from build123d import *

# Parameters (mm, degrees)
SKETCH1_R                  = 75
BOSS_EXTRUDE1_DEPTH        = 5
SKETCH2_R                  = 75
SKETCH2_R_2                = 73
BOSS_EXTRUDE2_DEPTH        = 60
BOSS_EXTRUDE3_START        = -60
BOSS_EXTRUDE3_DEPTH        = 60
F_10_0MM_DOWEL_HOLE1_D     = 10
F_10_0MM_DOWEL_HOLE1_DEPTH = 5
F_10_0MM_DOWEL_HOLE1_TIP   = 3.004303095
CUT_EXTRUDE1_REACH         = 173.61
CUT_EXTRUDE1_END_RADIUS    = 75
SKETCH7_W                  = 66.452990904
SKETCH7_H                  = 16
CUT_EXTRUDE2_START         = -39
CUT_EXTRUDE2_DEPTH         = 39


with BuildPart() as part:
    # Sketch1 → Boss-Extrude1 (new body)
    with BuildSketch(Plane(origin=(0, 0, 0), x_dir=(1, 0, 0), z_dir=(0, 1, 0))):
        with Locations(Location((0, 0, 0), (0, 0, 270))):
            Circle(SKETCH1_R)
    extrude(amount=BOSS_EXTRUDE1_DEPTH)

    # Sketch2 → Boss-Extrude2 (add)
    with BuildSketch(Plane(origin=(0, 5, 0), x_dir=(1, 0, 0), z_dir=(0, 1, 0))):
        with Locations(Location((0, 0, 0), (0, 0, 270))):
            Circle(SKETCH2_R)
        with Locations(Location((0, 0, 0), (0, 0, 270))):
            Circle(SKETCH2_R_2, mode=Mode.SUBTRACT)
    extrude(amount=BOSS_EXTRUDE2_DEPTH)

    # Sketch3 → Boss-Extrude3 (add)
    with BuildSketch(Plane(origin=(0, 65, 0), x_dir=(1, 0, 0), z_dir=(0, 1, 0)).offset(BOSS_EXTRUDE3_START)):
        with BuildLine():
            ThreePointArc((26.551836095, 68), (0, 73), (-26.551836095, 68))
            Line((-26.551836095, 68), (26.551836095, 68))
        make_face()
        with BuildLine():
            ThreePointArc((31.638584039, 68), (0, 75), (-31.638584039, 68))
            Line((-31.638584039, 68), (-26.551836095, 68))
            ThreePointArc((-26.551836095, 68), (0, 73), (26.551836095, 68))
            Line((26.551836095, 68), (31.638584039, 68))
        make_face()
        with BuildLine():
            Line((-33.226495452, -65), (-37.416573868, -65))
            ThreePointArc((-37.416573868, -65), (0, -75), (37.416573868, -65))
            Line((37.416573868, -65), (33.226495452, -65))
            ThreePointArc((33.226495452, -65), (0, -73), (-33.226495452, -65))
        make_face()
        with BuildLine():
            Line((33.226495452, -65), (-33.226495452, -65))
            ThreePointArc((-33.226495452, -65), (0, -73), (33.226495452, -65))
        make_face()
    extrude(amount=BOSS_EXTRUDE3_DEPTH)

    # Ø10.0mm Dowel Hole1
    with Locations(Plane(origin=(0, 5, 0), x_dir=(1, 0, 0), z_dir=(0, 1, 0))):
        with Locations((0, 0)):
            Hole(F_10_0MM_DOWEL_HOLE1_D / 2, depth=F_10_0MM_DOWEL_HOLE1_DEPTH)
            with Locations((0, 0, -(F_10_0MM_DOWEL_HOLE1_DEPTH + F_10_0MM_DOWEL_HOLE1_TIP / 2))):  # 118° drill point
                Cone(0, F_10_0MM_DOWEL_HOLE1_D / 2, F_10_0MM_DOWEL_HOLE1_TIP, mode=Mode.SUBTRACT)

    # Cut-Extrude1: up to this cylinder (the profile starts inside it)
    cut_extrude1_end = Plane(origin=(0, 57, 0), z_dir=(0, -1, 0)) * Cylinder(CUT_EXTRUDE1_END_RADIUS, 498.22, mode=Mode.PRIVATE)
    # Sketch7 → Cut-Extrude1 (cut, up to the surface)
    with BuildSketch(Plane(origin=(0, 0, 65), x_dir=(-1, 0, 0), z_dir=(0, 0, -1)), mode=Mode.PRIVATE) as cut_extrude1_sk1:
        with Locations((0, 57)):
            Rectangle(SKETCH7_W, SKETCH7_H)
    cut_extrude1_tool1 = extrude(cut_extrude1_sk1.sketch, amount=-CUT_EXTRUDE1_REACH, mode=Mode.PRIVATE) & cut_extrude1_end
    add(cut_extrude1_tool1.solids().sort_by_distance((0, 57, 65))[0], mode=Mode.SUBTRACT)

    # Sketch8 → Cut-Extrude2 (cut)
    with BuildSketch(Plane(origin=(0, 49, 0), x_dir=(1, 0, 0), z_dir=(0, 1, 0)).offset(CUT_EXTRUDE2_START)):
        with BuildLine():
            Line((-33.226495452, -67.238381896), (33.226495452, -67.238381896))
            ThreePointArc((33.226495452, -67.238381896), (0, -75), (-33.226495452, -67.238381896))
        make_face()
    extrude(amount=CUT_EXTRUDE2_DEPTH, mode=Mode.SUBTRACT)


solid = part.part
The listing builds one solid part. Answer for the finished solid, in the listing's coordinates (mm). A direction names the side the tool comes from. Coordinates: 2 decimals unless noted, no trailing zeros. Write each loop counter-clockwise with the first axis right and the second up, starting at its lowest first coordinate (ties: lowest second). Pieces come first, ordered by that corner, then holes. Notation, with made-up numbers: M 73.25,-31 L 97.25,-31 A22 cw 97.25,-7 Z; hole C 69.25,61.5 d6. An arc over 180 degrees is marked long. Write each question's results on one line, items separated by ' | '.
Item 1: The part is cut by section B-B on z = 0. Determine the outline of the cut face in (x, y), and give its area (3 significant figures).
Answer below:
outline: M -75,0 L -5,0 L -5,5 L -73,5 L -73,65 L -75,65 Z; M 5,0 L 75,0 L 75,65 L 73,65 L 73,5 L 5,5 Z | area: 940 mm2
Item 2: Consider probe 1 along Y at (x, z) = (-32, 22); probe 2 along Z at (x, y) = (-1.5, 21) (3 decimals); probe 3 along Z at (x, y) = (-44, 54). Determine where each line is inside the solid, lowest interval first. Write a range as [from, to].
Answer below:
probe 1: [0, 5] | probe 2: [-74.985, -68], [65, 67.238] | probe 3: [-60.74, -58.25], [58.25, 60.74]
Item 3: The part is cut by section A-A on x = 0. Determine the outline of the cut face in (y, z).
Answer below:
outline: M 0,-75 L 65,-75 L 65,-68 L 5,-68 L 5,-5 L 0,-5 Z; M 0,5 L 5,5 L 5,65 L 49,65 L 49,67.24 L 10,67.24 L 10,75 L 0,75 Z
Item 4: For a pull along X with two mould halves and no side action, classify faces 4 (the face through (0, 35, -68)), 5 (the face through (3.298, 32.045, -74.927)), 6 (the face through (1.08, 2.46, 4.88)), 7 (the face through (0, 65, -73)) as released by +X, released by -X, zero draft, split by the parting line, or undercut.
Answer below:
face 4: undercut | face 5: split by the parting line | face 6: undercut | face 7: zero draft
Item 5: The part is cut by section D-D on x = -45. Determine the outline of the cut face in (y, z).
Answer below:
outline: M 0,-60 L 65,-60 L 65,-57.48 L 5,-57.48 L 5,57.48 L 65,57.48 L 65,60 L 0,60 Z
Item 6: The part is cut by section C-C on y = 36. Determine the outline of the cut face in (x, z), and give its area (3 significant figures).
Answer below:
outline: M -33.23,67.24 A75 ccw long 33.23,67.24 Z; hole M -33.23,65 A73 ccw -26.55,-68 L 26.55,-68 A73 ccw 33.23,65 Z | area: 1,120 mm2
Item 7: Given P1, Ø2.5, axis at y = 57.5, z = 66, coming from the +X side; P2, Ø6, axis at y = 54, z = -2.5, coming from the -X side; P3, Ø2.5, axis at y = 55, z = 66.5, coming from the -X side; P4, Ø2.5, axis at x = 9.5, z = 66, coming from the +Y side, each flat-ended and moving along its own axis, determine where each tip first touches the part or whether it passes through.
Answer below:
P1: x = 37.85 | P2: x = -75 | P3: x = -36.98 | P4: y = 49
Item 8: Which of the six approach directions +Z, -Z, +X, -X, +Y, -Y give full straight-line access (tool end or side, diameter ignored) to faces 1 (the face through (0, 10, 70)), 2 (the face through (-16, 0, -1)), 3 (the face through (1, 5, 12))?
Answer below:
face 1: +Z, +X, -X, +Y | face 2: +Z, -Z, +X, -X, -Y | face 3: +Y
